Read the model definition and answer for the solid it produces. Units are mm, in the model's axes. Face numbers are marked on the shaded views. Round coordinates to 2 decimals unless told otherwise and drop trailing zeros. Order: outer loops, then holes, each group sorted by start corner. A loop starts at its lowest first (then second) coordinate and runs counter-clockwise, first axis right, second up. Notation, with made-up numbers: (-26, 54.25) -> (-7, 54.25) arc R25 ccw to (-7, 83.25) -> close; hole circle Ø5 at (33.25, 49.25). An arc over 180 degrees is marked (long way). One line per item, written item: value. Start each with the question number.
1. Flat-ended cylindrical pins translate along their axes: pin 1 Ø1 at (x, y) = (4.5, 3.5) entering from +Z; pin 2 Ø1.7 at (x, z) = (-38.89, 16.11) entering from +Y; pin 3 Ø1.5 at (x, y) = (-15, 0.5) entering from +Z; pin 4 Ø4 at (y, z) = (2, 17) entering from -X. Find the tip coordinate at first contact, or state that the pin passes through.
2. Section A-A (z = 19) is taken. Give the vertices of the cut face in (x, y), then the cut area to 3 significant figures.
3. The mould has two halves that part along Z. Classify the marked faces 1, 2 and 3: released by +Z, released by -Z, zero draft, split by the parting line, or undercut.
4. Consider line 1 (Z direction, x = 0, y = 5); line 2 (X direction, y = 1.5, z = 38.5); line 3 (Z direction, x = 0, y = 3). Determine where each line is inside the solid, lowest interval first.
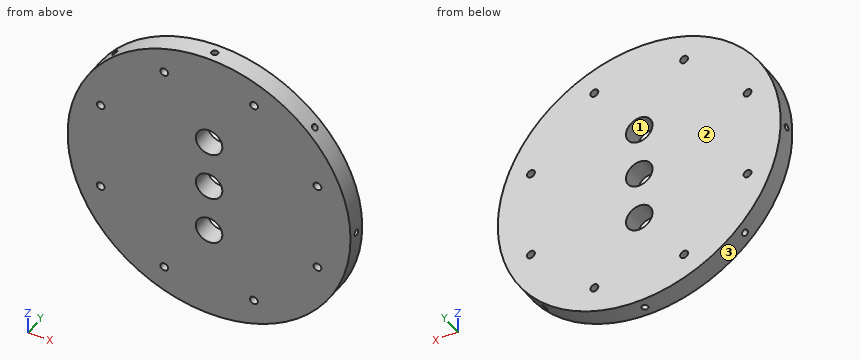
from build123d import *

# Parameters (mm, degrees)
SKETCH1_R                      = 50.8
BOSS_EXTRUDE1_DEPTH            = 7.112
SKETCH2_R                      = 4.7625
CUT_EXTRUDE1_DEPTH             = 8.112
F_4_40_TAPPED_HOLE1_AT_2_COUNT = 2
F_4_40_TAPPED_HOLE1_AT_2_PITCH = 18.336817374
CIRPATTERN7_COUNT              = 8
SKETCH11_R                     = 1.41224
CUT_EXTRUDE3_DEPTH             = 8.1120001
CIRPATTERN8_COUNT              = 8


with BuildPart() as part:
    # Sketch1 → Boss-Extrude1 (new body)
    with BuildSketch(Plane(origin=(0, 0, 0), x_dir=(1, 0, 0), z_dir=(0, 1, 0))):
        Circle(SKETCH1_R)
    extrude(amount=BOSS_EXTRUDE1_DEPTH)

    # Sketch2 → Cut-Extrude1 (cut, through all)
    with BuildSketch(Plane.XZ):
        Circle(SKETCH2_R)
        with Locations((0, -17.526)):
            Circle(SKETCH2_R)
        with Locations((0, 17.526)):
            Circle(SKETCH2_R)
    extrude(amount=-CUT_EXTRUDE1_DEPTH, mode=Mode.SUBTRACT)

    # Sketch8 → #4-40 Tapped Hole1 (revolve, cut)
    with BuildSketch(Plane(origin=(-0.062175227, 3.554407485, 50.799961951), x_dir=(0.999999251, 0, 0.001223922), z_dir=(0, 1, 0))):
        Polygon((0, 0), (0, 10.204152758), (1.1303, 9.525), (1.1303, 0), align=None)
    f_4_40_tapped_hole1 = revolve(axis=Axis((-0.062175227, 3.554407485, 50.799961951), (0.001223922, 0, -0.999999251)), mode=Mode.SUBTRACT)

    # #4-40 Tapped Hole1 at 2: #4-40 Tapped Hole1 ×2
    with Locations(*[Vector(0.92843035, 0.371504769, 0.001136327) * (i * F_4_40_TAPPED_HOLE1_AT_2_PITCH) for i in range(1, F_4_40_TAPPED_HOLE1_AT_2_COUNT)]):
        add(f_4_40_tapped_hole1, mode=Mode.SUBTRACT)

    # CirPattern7: #4-40 Tapped Hole1 ×8 about axis
    cirpattern7_axis = Axis((0, 7.112, 0), (0, 1, 0))
    for i in range(1, CIRPATTERN7_COUNT):
        add(f_4_40_tapped_hole1.rotate(cirpattern7_axis, i * 360 / CIRPATTERN7_COUNT), mode=Mode.SUBTRACT)

    # CirPattern7 copy 1 sketch → CirPattern7 copy 1 (revolve, cut)
    with BuildSketch(Plane(origin=(47.92987631, 10.366622592, 23.941586281), x_dir=(0.707971695, 0, -0.706240808), z_dir=(0, 1, 0))):
        Polygon((0, 0), (0, 10.204152758), (1.1303, 9.525), (1.1303, 0), align=None)
    revolve(axis=Axis((47.92987631, 10.366622592, 23.941586281), (-0.706240808, 0, -0.707971695)), mode=Mode.SUBTRACT)

    # CirPattern7 copy 2 sketch → CirPattern7 copy 2 (revolve, cut)
    with BuildSketch(Plane(origin=(50.820798572, 10.366622592, -16.962282549), x_dir=(0.001223922, 0, -0.999999251), z_dir=(0, 1, 0))):
        Polygon((0, 0), (0, 10.204152758), (1.1303, 9.525), (1.1303, 0), align=None)
    revolve(axis=Axis((50.820798572, 10.366622592, -16.962282549), (-0.999999251, 0, -0.001223922)), mode=Mode.SUBTRACT)

    # CirPattern7 copy 3 sketch → CirPattern7 copy 3 (revolve, cut)
    with BuildSketch(Plane(origin=(23.941586281, 10.366622592, -47.92987631), x_dir=(-0.706240808, 0, -0.707971695), z_dir=(0, 1, 0))):
        Polygon((0, 0), (0, 10.204152758), (1.1303, 9.525), (1.1303, 0), align=None)
    revolve(axis=Axis((23.941586281, 10.366622592, -47.92987631), (-0.707971695, 0, 0.706240808)), mode=Mode.SUBTRACT)

    # CirPattern7 copy 4 sketch → CirPattern7 copy 4 (revolve, cut)
    with BuildSketch(Plane(origin=(-16.962282549, 10.366622592, -50.820798572), x_dir=(-0.999999251, 0, -0.001223922), z_dir=(0, 1, 0))):
        Polygon((0, 0), (0, 10.204152758), (1.1303, 9.525), (1.1303, 0), align=None)
    revolve(axis=Axis((-16.962282549, 10.366622592, -50.820798572), (-0.001223922, 0, 0.999999251)), mode=Mode.SUBTRACT)

    # CirPattern7 copy 5 sketch → CirPattern7 copy 5 (revolve, cut)
    with BuildSketch(Plane(origin=(-47.92987631, 10.366622592, -23.941586281), x_dir=(-0.707971695, 0, 0.706240808), z_dir=(0, 1, 0))):
        Polygon((0, 0), (0, 10.204152758), (1.1303, 9.525), (1.1303, 0), align=None)
    revolve(axis=Axis((-47.92987631, 10.366622592, -23.941586281), (0.706240808, 0, 0.707971695)), mode=Mode.SUBTRACT)

    # CirPattern7 copy 6 sketch → CirPattern7 copy 6 (revolve, cut)
    with BuildSketch(Plane(origin=(-50.820798572, 10.366622592, 16.962282549), x_dir=(-0.001223922, 0, 0.999999251), z_dir=(0, 1, 0))):
        Polygon((0, 0), (0, 10.204152758), (1.1303, 9.525), (1.1303, 0), align=None)
    revolve(axis=Axis((-50.820798572, 10.366622592, 16.962282549), (0.999999251, 0, 0.001223922)), mode=Mode.SUBTRACT)

    # CirPattern7 copy 7 sketch → CirPattern7 copy 7 (revolve, cut)
    with BuildSketch(Plane(origin=(-23.941586281, 10.366622592, 47.92987631), x_dir=(0.706240808, 0, 0.707971695), z_dir=(0, 1, 0))):
        Polygon((0, 0), (0, 10.204152758), (1.1303, 9.525), (1.1303, 0), align=None)
    revolve(axis=Axis((-23.941586281, 10.366622592, 47.92987631), (0.707971695, 0, -0.706240808)), mode=Mode.SUBTRACT)

    # Sketch11 → Cut-Extrude3 (cut, through all)
    with BuildSketch(Plane(origin=(0, 7.112, 0), x_dir=(1, 0, 0), z_dir=(0, 1, 0))):
        with Locations((-38.892386202, 16.109753838)):
            Circle(SKETCH11_R)
    cut_extrude3 = extrude(amount=-CUT_EXTRUDE3_DEPTH, mode=Mode.SUBTRACT)

    # CirPattern8: Cut-Extrude3 ×8 about axis
    cirpattern8_axis = Axis((0, 0, 0), (0, 1, 0))
    for i in range(1, CIRPATTERN8_COUNT):
        add(cut_extrude3.rotate(cirpattern8_axis, i * 360 / CIRPATTERN8_COUNT), mode=Mode.SUBTRACT)


solid = part.part
Answer:
1. pin 1: z = 50.64
1. pin 2: through
1. pin 3: z = 48.76
1. pin 4: x = -48.53
2. outline: (-47.11, 0) -> (-4.53, 0) -> (-4.53, 7.11) -> (-47.11, 7.11) -> close; (4.53, 0) -> (47.11, 0) -> (47.11, 7.11) -> (4.53, 7.11) -> close
2. area: 606 mm^2
3. face 1: undercut
3. face 2: zero draft
3. face 3: split by the parting line
4. line 1: -50.8 to -22.29, -12.76 to -4.76, 4.76 to 12.76, 22.29 to 50.8
4. line 2: -33.14 to -17.47, -14.75 to 14.75, 17.47 to 33.14
4. line 3: -40.93 to -22.29, -12.76 to -4.76, 4.76 to 12.76, 22.29 to 40.93
